Input: dimensioned drawing with shaded views. Units: mm. Origin: part minimum x, y, z. A direction names the side the tool comes from. Round coordinates to 2 decimals unless told otherwise and drop trailing zeros. Order: outer loops, then holes, each group sorted by start corner. A loop starts at its lowest first (then second) coordinate and runs counter-clockwise, first axis right, second up.
Item 1: Cut plane B-B on x = 38.1. Output: boundary loops of the cut face in (y, z).
Item 2: Cut plane A-A on y = 25.4. Output: boundary loops of the cut face in (x, z).
Item 3: Mould query, pull axis Y, two halves, no side actions, for the marked faces 4, 5 and 6. Classes: released by +Y, released by -Y, zero draft, split by the parting line, or undercut.
Item 4: Line query: L1, parallel to X at y = 25.4, z = 7; L2, parallel to Y at x = 38.1, z = 6.5; L3, parallel to X at y = 39, z = 12.25. Output: solid intervals per line, ascending.
Item 5: Reachability of the marked faces 1, 2 and 3 from +Z, -Z, +X, -X, +Y, -Y: full face, straight path, thin tool, end or side. Return the list, or none.
Item 6: Cut plane C-C on z = 4.5. Output: boundary loops of the cut face in (x, y), then the cut area to 3 significant figures.
Item 7: First-contact query: pin 1 (5 mm diameter, centred on x = 36.5, y = 42.5, fed in from +Z); pin 2 (5.5 mm diameter, centred on x = 67, y = 31.5, fed in from +Z); pin 3 (15 mm diameter, centred on x = 38.1, y = 25.4, fed in from -Z). Flat tips, straight axial feed; report the tip coordinate or a pass-through.
Item 8: Cut plane D-D on y = 17.5. Output: boundary loops of the cut face in (x, z).
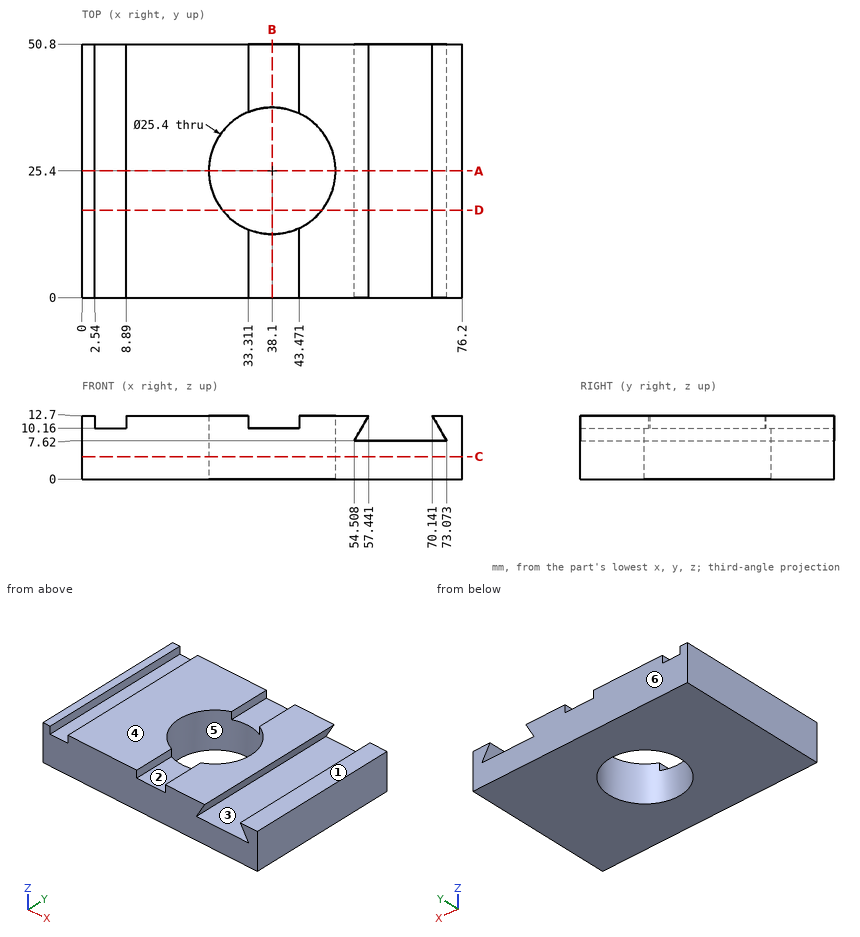
From the geometry:
1. outline: (0, 0) - (12.7, 0) - (12.7, 10.16) - (0, 10.16) - close; (38.1, 0) - (50.8, 0) - (50.8, 10.16) - (38.1, 10.16) - close
2. outline: (0, 0) - (25.4, 0) - (25.4, 12.7) - (8.89, 12.7) - (8.89, 10.16) - (2.54, 10.16) - (2.54, 12.7) - (0, 12.7) - close; (50.8, 0) - (76.2, 0) - (76.2, 12.7) - (70.14, 12.7) - (73.07, 7.62) - (54.51, 7.62) - (57.44, 12.7) - (50.8, 12.7) - close
3. face 4: zero draft
3. face 5: undercut
3. face 6: released by +Y
4. L1: x = 0 to 25.4, 50.8 to 76.2
4. L2: y = 0 to 12.7, 38.1 to 50.8
4. L3: x = 0 to 2.54, 8.89 to 33.31, 43.47 to 57.18, 70.4 to 76.2
5. face 1: +Z, +X, -X, +Y, -Y
5. face 2: +Z, +Y, -Y
5. face 3: +Y, -Y
6. outline: (0, 0) - (76.2, 0) - (76.2, 50.8) - (0, 50.8) - close; hole circle Ø25.4 at (38.1, 25.4)
6. area: 3,360 mm2
7. pin 1: stops at z = 10.16
7. pin 2: stops at z = 7.62
7. pin 3: passes through
8. outline: (0, 0) - (28.16, 0) - (28.16, 12.7) - (8.89, 12.7) - (8.89, 10.16) - (2.54, 10.16) - (2.54, 12.7) - (0, 12.7) - close; (48.04, 0) - (76.2, 0) - (76.2, 12.7) - (70.14, 12.7) - (73.07, 7.62) - (54.51, 7.62) - (57.44, 12.7) - (48.04, 12.7) - close
